from build123d import *

# Parameters (mm, degrees)
F1_DEPTH      = 40
F1_DEPTH_BACK = 40
F2_DEPTH      = 5
F2_DEPTH_BACK = 5
F0_R          = 25
F3_DEPTH      = 30
F3_DEPTH_BACK = 30
F4_R          = 5
F5_DEPTH      = 25


with BuildPart() as f1:
    # F0 (on Front) → F1 (new body, two sides)
    with BuildSketch(Plane.XZ) as f1_sk:
        Polygon((-18.003343, -13.36493), (-48.003343, -13.36493), (-48.003343, -28.36493), (-18.003343, -28.36493), (-18.003343, -23.36493), (41.996657, -23.36493), (41.996657, -28.36493), (71.996657, -28.36493), (71.996657, -13.36493), (46.996657, -13.36493), (41.996657, -13.36493), (36.996657, -13.36493), align=None)
    extrude(amount=F1_DEPTH)
    extrude(f1_sk.sketch, amount=-F1_DEPTH_BACK)

    # F0 (on Front) → F2 (join, two sides)
    with BuildSketch(Plane.XZ) as f2_sk:
        with BuildLine():
            Line((6.996657, 46.63507), (-18.003343, -13.36493))
            Line((-18.003343, -13.36493), (36.996657, -13.36493))
            Line((36.996657, -13.36493), (36.996657, 11.994054))
            ThreePointArc((36.996657, 11.994054), (15.539144, 23.722191), (6.996657, 46.63507))
        make_face()
    extrude(amount=F2_DEPTH)
    extrude(f2_sk.sketch, amount=-F2_DEPTH_BACK)

    # F0 (on Front) → F3 (join, two sides)
    with BuildSketch(Plane.XZ) as f3_sk:
        with BuildLine():
            ThreePointArc((76.996657, 46.63507), (41.996657, 81.63507), (6.996657, 46.63507))
            ThreePointArc((6.996657, 46.63507), (15.539144, 23.722191), (36.996657, 11.994054))
            ThreePointArc((36.996657, 11.994054), (41.996657, 11.63507), (46.996657, 11.994054))
            ThreePointArc((46.996657, 11.994054), (68.45417, 23.722191), (76.996657, 46.63507))
        make_face()
        with Locations((41.996657, 46.63507)):
            Circle(F0_R, mode=Mode.SUBTRACT)
        with BuildLine():
            Line((36.996657, 11.994054), (36.996657, -13.36493))
            Line((36.996657, -13.36493), (41.996657, -13.36493))
            Line((41.996657, -13.36493), (46.996657, -13.36493))
            Line((46.996657, -13.36493), (46.996657, 11.994054))
            ThreePointArc((46.996657, 11.994054), (41.996657, 11.63507), (36.996657, 11.994054))
        make_face()
    extrude(amount=F3_DEPTH)
    extrude(f3_sk.sketch, amount=-F3_DEPTH_BACK)

    # F4 (on face) → F5 (cut)
    with BuildSketch(Plane.XY.offset(-13.36493)):
        with BuildLine():
            ThreePointArc((-33.003343, -30), (-29.467809, -28.535534), (-28.003343, -25))
            ThreePointArc((-28.003343, -25), (-36.538877, -21.464466), (-33.003343, -30))
        make_face()
        with BuildLine():
            ThreePointArc((-33.003343, 30), (-36.538877, 21.464466), (-28.003343, 25))
            ThreePointArc((-28.003343, 25), (-29.467809, 28.535534), (-33.003343, 30))
        make_face()
        with Locations((33.003343, 25)):
            Circle(F4_R)
        with Locations((56.996657, -25)):
            Circle(F4_R)
        with Locations((56.996657, 25)):
            Circle(F4_R)
    extrude(amount=-F5_DEPTH, mode=Mode.SUBTRACT)


solid = f1.part
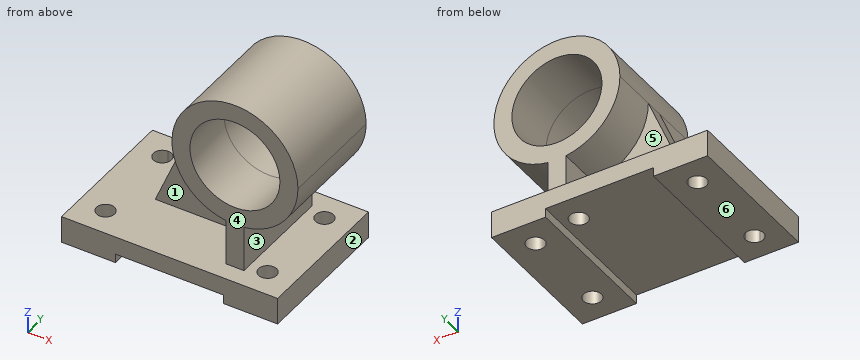
Here's how the part is built. I have some questions about the finished solid (model axes, mm). Face numbers are marked on the shaded views. A direction names the side the tool comes from. Coordinates: 2 decimals unless noted, no trailing zeros. Order: outer loops, then holes, each group sorted by start corner. A loop starts at its lowest first (then second) coordinate and runs counter-clockwise, first axis right, second up. Notation, with made-up numbers: (59, 38.5) - (77, 38.5) arc R21 cw to (77, 60.5) - close; hole circle Ø2 at (81.25, -25). An arc over 180 degrees is marked (long way). Use CSV: the item, a comma, the result in double quotes. Start each with the question number.
1. For the marked faces 1, 2 and 3, which set-ups out of +Z, -Z, +X, -X, +Y, -Y let a thin tool reach every point of the face, with its end or its side?
2. If we mould it in two halves opening along Y, with no side actions, what happens to the marked faces 4, 5 and 6? For each: +Y half, -Y half, draft (parallel to the pull), parting line (faces both ways), or undercut.
3. Suppose I cut it at C-C on y = 17. List the corners of the cut face in (x, z) for me.
4. Suppose I cut it at B-B on x = 30.5. List the corners of the cut face in (y, z) for me.
5. Suppose I cut it at D-D on x = -1.5. List the corners of the cut face in (y, z) for me, then the cut area to 3 significant figures.
6. Suppose I cut it at A-A on y = 26.5. List the corners of the cut face in (x, z) for me.
7. I'm going to push flat-ended pins straight in: pin 1 (1 mm diameter, centred on y = -26, z = 9.5, fed in from +X); pin 2 (2 mm diameter, centred on y = -24, z = 52.5, fed in from +X); pin 3 (6 mm diameter, centred on x = 36, z = 18, fed in from +Y); pin 4 (8 mm diameter, centred on x = -33, y = 25, fed in from -Z). Where does each tip first touch, or does it pass through?
8. Please list where these lines run through material, in increasing order: line 1 (Z direction, x = 59.5, y = 1.5); line 2 (Z direction, x = 62.5, y = 7); line 3 (Y direction, x = 3.5, z = 23). Write a range as from..to.
Output:
1,face 1,"-X, -Y"
1,face 2,"-Z, +X, +Y, -Y"
1,face 3,"+X, +Y, -Y"
2,face 4,"-Y half"
2,face 5,"+Y half"
2,face 6,"draft"
3,outline,"(-48, -28.36) - (-18, -28.36) - (-18, -23.36) - (42, -23.36) - (42, -28.36) - (72, -28.36) - (72, -13.36) - (47, -13.36) - (47, 11.99) arc R35 ccw to (77, 46.64) arc R35 ccw to (7, 46.64) arc R35 ccw to (37, 11.99) - (37, -13.36) - (-48, -13.36) - close; hole circle Ø50 at (42, 46.64)"
4,outline,"(-40, -23.36) - (20.67, -23.36) - (20.67, -13.36) - (5, -13.36) - (5, 13.58) - (30, 13.58) - (30, 24.44) - (-30, 24.44) - (-30, 13.58) - (-5, 13.58) - (-5, -13.36) - (-40, -13.36) - close; (-30, 68.83) - (30, 68.83) - (30, 79.69) - (-30, 79.69) - close; (29.33, -23.36) - (40, -23.36) - (40, -13.36) - (29.33, -13.36) - close"
5,outline,"(-40, -23.36) - (40, -23.36) - (40, -13.36) - (5, -13.36) - (5, 26.24) - (-5, 26.24) - (-5, -13.36) - (-40, -13.36) - close"
5,area,"1,200 mm2"
6,outline,"(-48, -28.36) - (-37.77, -28.36) - (-37.77, -13.36) - (-48, -13.36) - close; (-28.23, -28.36) - (-18, -28.36) - (-18, -23.36) - (28.23, -23.36) - (28.23, -13.36) - (-28.23, -13.36) - close; (7, 46.64) arc R35 ccw to (37, 11.99) - (37, -13.36) - (37.77, -13.36) - (37.77, -23.36) - (42, -23.36) - (42, -28.36) - (52.23, -28.36) - (52.23, -13.36) - (47, -13.36) - (47, 11.99) arc R35 ccw to (77, 46.64) arc R35 ccw to start; (61.77, -28.36) - (72, -28.36) - (72, -13.36) - (61.77, -13.36) - close; hole circle Ø50 at (42, 46.64)"
7,pin 1,"stops at x = 47"
7,pin 2,"stops at x = 76.66"
7,pin 3,"stops at y = 30"
7,pin 4,"passes through"
8,line 1,"z = -28.36..-13.36, 16.33..28.78, 64.49..76.94"
8,line 2,"z = -28.36..-13.36, 18.27..32.33, 60.94..75"
8,line 3,"y = -5..5"
